from build123d import *

# Parameters (mm, degrees)
SKETCH2_W                                   = 101.6
SKETCH2_H                                   = 127
BOSS_EXTRUDE1_DEPTH                         = 3.175
SKETCH5_R                                   = 3.9751
CUT_EXTRUDE1_DEPTH                          = 3.175
BOSS_EXTRUDE3_DEPTH                         = 92.87256
BOSS_EXTRUDE4_DEPTH                         = 6.35
SKETCH18_R                                  = 3.175
CUT_EXTRUDE3_DEPTH                          = 6.8072
FILLET4_R                                   = 4.0005
CUT_EXTRUDE4_DEPTH                          = 34.5948
CUT_EXTRUDE5_DEPTH                          = 2.9972
FILLET7_R                                   = 6.35
CSK_FOR_1_4_FLAT_HEAD_MACHINE_SCREW_2_COUNT = 2
CSK_FOR_1_4_FLAT_HEAD_MACHINE_SCREW_2_PITCH = 55.9
SKETCH36_R                                  = 6.4389
CUT_EXTRUDE6_DEPTH                          = 2.54


with BuildPart() as part:
    # Sketch2 → Boss-Extrude1 (new body)
    with BuildSketch(Plane.XY):
        with Locations((50.8, 63.5)):
            Rectangle(SKETCH2_W, SKETCH2_H)
    extrude(amount=BOSS_EXTRUDE1_DEPTH)

    # Sketch5 → Cut-Extrude1 (cut)
    with BuildSketch(Plane(origin=(0, 0, 0), x_dir=(-1, 0, 0), z_dir=(0, 0, -1))):
        with BuildLine():
            Line((-81.586228812, 65.152573183), (-58.571239337, 65.152573183))
            ThreePointArc((-58.571239337, 65.152573183), (-49.65943867, 58.729036089), (-53.287760408, 48.359981104))
            ThreePointArc((-53.287760408, 48.359981104), (-57.249364207, 28.049269577), (-36.93865268, 24.087665778))
            ThreePointArc((-36.93865268, 24.087665778), (-28.337713232, 24.971703827), (-22.817162059, 18.317291951))
            ThreePointArc((-22.817162059, 18.317291951), (-16.509170131, 7.896881921), (-5.03428, 3.81))
            Line((-5.03428, 3.81), (-5.03428, 0))
            Line((-5.03428, 0), (0, 0))
            Line((0, 0), (0, 127))
            Line((0, 127), (-101.6, 127))
            Line((-101.6, 127), (-101.6, 0))
            Line((-101.6, 0), (-97.90684, 0))
            Line((-97.90684, 0), (-97.90684, 65.152573183))
            Line((-97.90684, 65.152573183), (-81.586228812, 65.152573183))
        make_face()
        with Locations((-58.416247506, 55.973867932)):
            Circle(SKETCH5_R)
        with Locations((-31.810165582, 16.473778949)):
            Circle(SKETCH5_R)
    extrude(amount=-CUT_EXTRUDE1_DEPTH, mode=Mode.SUBTRACT)

    # Sketch10 → Boss-Extrude3 (add)
    with BuildSketch(Plane(origin=(5.03428, 0, 0), x_dir=(0, 0, -1), z_dir=(1, 0, 0))):
        Polygon((-3.175, 0), (-4.2418, 0), (-4.2418, -2.9972), (-34.5948, -2.9972), (-34.5948, 0), (-34.5948, 3.81), (-3.175, 3.81), align=None)
    extrude(amount=BOSS_EXTRUDE3_DEPTH)

    # Sketch11 → Boss-Extrude4 (add)
    with BuildSketch(Plane(origin=(97.90684, 0, 0), x_dir=(0, 0, -1), z_dir=(1, 0, 0))):
        Polygon((-3.175, 65.152573183), (-3.175, 3.81), (-34.5948, 3.81), align=None)
    extrude(amount=-BOSS_EXTRUDE4_DEPTH)

    # Sketch18 → Cut-Extrude3 (cut)
    with BuildSketch(Plane.XZ.offset(2.9972)):
        with Locations(Location((25.968032816, 23.228300068, 0), (0, 0, 270))):
            Circle(SKETCH18_R)
        with Locations(Location((81.868032816, 23.228300068, 0), (0, 0, 270))):
            Circle(SKETCH18_R)
    extrude(amount=-CUT_EXTRUDE3_DEPTH, mode=Mode.SUBTRACT)

    # Fillet4
    fillet4_edges = [part.edges().sort_by_distance(p)[0] for p in [
        (97.90684, -1.4986, 4.2418),
        (5.03428, -1.4986, 4.2418),
        (97.90684, 0.4064, 34.5948),
        (5.03428, 0.4064, 34.5948),
    ]]
    fillet(fillet4_edges, radius=FILLET4_R)

    # Mirror5: part across plane


with BuildPart() as part_1:
    add(part.part)
    add(part.part.mirror(Plane.XY))

    # Sketch25 → Cut-Extrude4 (cut)
    with BuildSketch(Plane.XY):
        Polygon((105.475480197, -15.241589329), (106.840773124, 71.833759528), (-8.541984089, 73.642896836), (-9.907277015, -13.432452021), align=None)
    extrude(amount=CUT_EXTRUDE4_DEPTH, mode=Mode.SUBTRACT)

    # Sketch28 → Cut-Extrude5 (cut)
    with BuildSketch(Plane.XZ.offset(2.9972)):
        with BuildLine():
            Line((93.90634, -4.2418), (9.03478, -4.2418))
            ThreePointArc((9.03478, -4.2418), (6.205999322, -5.413519322), (5.03428, -8.2423))
            Line((5.03428, -8.2423), (5.03428, -30.5943))
            ThreePointArc((5.03428, -30.5943), (6.205999322, -33.423080678), (9.03478, -34.5948))
            Line((9.03478, -34.5948), (93.90634, -34.5948))
            ThreePointArc((93.90634, -34.5948), (96.735120678, -33.423080678), (97.90684, -30.5943))
            Line((97.90684, -30.5943), (97.90684, -8.2423))
            ThreePointArc((97.90684, -8.2423), (96.735120678, -5.413519322), (93.90634, -4.2418))
        make_face()
    extrude(amount=-CUT_EXTRUDE5_DEPTH, mode=Mode.SUBTRACT)

    # Fillet7
    fillet7_edges = [part_1.edges().sort_by_distance(p)[0] for p in [
        (91.55684, 3.81, -18.8849),
    ]]
    fillet(fillet7_edges, radius=FILLET7_R)

    # Sketch35 → CSK for 1/4 Flat Head Machine Screw (100)1 (revolve, cut)
    with BuildSketch(Plane(origin=(25.968032816, 3.81, -23.228300068), x_dir=(0, 0, 1), z_dir=(1, 0, 0))):
        Polygon((0, 0), (0, 3.81), (3.57124, 3.81), (3.57124, 3.298865467), (6.4389, 0), align=None)
    csk_for_1_4_flat_head_machine_screw_100 = revolve(axis=Axis((25.968032816, 10.16, -23.228300068), (0, -1, 0)), mode=Mode.SUBTRACT)

    # CSK for 1_4 Flat Head Machine Screw  2: CSK for 1/4 Flat Head Machine Screw (100)1 ×2
    with Locations(*[(i * CSK_FOR_1_4_FLAT_HEAD_MACHINE_SCREW_2_PITCH, 0, 0) for i in range(1, CSK_FOR_1_4_FLAT_HEAD_MACHINE_SCREW_2_COUNT)]):
        add(csk_for_1_4_flat_head_machine_screw_100, mode=Mode.SUBTRACT)

    # Sketch36 → Cut-Extrude6 (cut)
    with BuildSketch(Plane(origin=(0, 3.81, 0), x_dir=(1, 0, 0), z_dir=(0, 1, 0))):
        with Locations((81.868032816, 23.228300068)):
            Circle(SKETCH36_R)
    extrude(amount=CUT_EXTRUDE6_DEPTH, mode=Mode.SUBTRACT)


solid = part_1.part
Could you check a few things on this model? Use its own coordinates, in mm. A direction names the side the tool comes from. Coordinates: 2 decimals unless noted, no trailing zeros. Write each loop counter-clockwise with the first axis right and the second up, starting at its lowest first coordinate (ties: lowest second). Pieces come first, ordered by that corner, then holes. Notation, with made-up numbers: M 14,-13.5 L 56,-13.5 A23 ccw 56,25.5 Z; hole C 38.25,37 d6. An arc over 180 degrees is marked long. One line per question, with ' | ' between items.
1) Imagine slicing it at C-C, the plane z = -8. Write out the boundary of the cut face in (x, y), and give its area (3 significant figures).
Checks:
outline: M 5.03,0 L 97.91,0 L 97.91,55.73 L 91.56,55.73 L 91.56,10.16 A6.35 cw 85.21,3.81 L 5.03,3.81 Z | area: 692 mm²
2) For faces 4 (the face through (88.306, 4.119, -23.136)), 5 (the face through (89.647, 5.621, -19.105)), 6 (the face through (97.907, 26, -12)), which set-ups out of +Z, -Z, +X, -X, +Y, -Y let a thin tool reach every point of the face, with its end or its side?
Checks:
face 4: -X, +Y | face 5: -Z, -X, +Y | face 6: +Z, -Z, +X, +Y, -Y
3) If we mould it in two halves opening along Z, with no side actions, what happens to faces 1 (the face through (97.16, 3.15, -32.92)), 2 (the face through (57.426, 28.318, -1.565)), 3 (the face through (29.136, 0.259, -21.58))? For each: released by +Z, released by -Z, zero draft, split by the parting line, or undercut.
Checks:
face 1: released by -Z | face 2: zero draft | face 3: undercut
4) Imagine slicing it at D-D, the plane x = 56.5. Write out the boundary of the cut face in (y, z) (3 decimals).
Checks:
outline: M 0,-34.595 L 3.81,-34.595 L 3.81,-3.175 L 27.034,-3.175 L 27.034,0 L 0,0 Z; M 45.414,-3.175 L 52.491,-3.175 L 52.491,0 L 45.414,0 Z; M 59.457,-3.175 L 64.952,-3.175 L 64.952,0 L 59.457,0 Z
5) For pin 1 Ø8 at (x, z) = (81.87, -23.23) entering from +Y; pin 2 Ø6 at (x, z) = (35, -10) entering from +Y; pin 3 Ø6 at (y, z) = (41, -16.5) entering from -X, each with a flat end and sliding along its axis, tell me the tip position at first contact or that it passes through.
Checks:
pin 1: y = 1.01 | pin 2: y = 3.81 | pin 3: x = 91.56
6) Imagine slicing it at B-B, the plane x = 34.5. Write out the boundary of the cut face in (y, z) (3 decimals), and give its area (3 significant figures).
Checks:
outline: M 0,-34.595 L 3.81,-34.595 L 3.81,-3.175 L 13.547,-3.175 L 13.547,0 L 0,0 Z; M 19.401,-3.175 L 25.251,-3.175 L 25.251,0 L 19.401,0 Z | area: 181 mm²
7) I need wall thicknesses on probe 1 along Y at (x, z) = (23, -13.5); probe 2 along X at (y, z) = (16.5, -2); probe 3 along Y at (x, z) = (32.5, -2). Which ranges of each line are inside material? Lowest first, please. Write a range as [from, to].
Checks:
probe 1: [0, 3.81] | probe 2: [22.35, 27.84], [35.79, 97.91] | probe 3: [0, 12.56], [20.39, 25.63]
8) Imagine slicing it at A-A, the plane y = 53. Write out the boundary of the cut face in (x, z) (3 decimals), and give its area (3 significant figures).
Checks:
outline: M 49.731,-3.175 L 55.779,-3.175 L 55.779,0 L 49.731,0 Z; M 61.054,-3.175 L 91.557,-3.175 L 91.557,-9.4 L 97.907,-9.4 L 97.907,0 L 61.054,0 Z | area: 176 mm²
